```python
from build123d import *

# Parameters (mm, degrees)
SKETCH_1_W          = 9
SKETCH_1_H          = 9
EXTRUDE_1_DEPTH     = 3
SKETCH_2_W          = 14
SKETCH_2_H          = 14
EXTRUDE_2_DEPTH     = 2.5
CHAMFER_1_SIZE      = 1.5
SKETCH_3_W          = 12
SKETCH_3_H          = 10.4
EXTRUDE_3_DEPTH     = 12
EXTRUDE_4_DEPTH     = 2.3
SKETCH_5_W          = 0.5
SKETCH_5_H          = 3
EXTRUDE_5_DEPTH     = 4
SKETCH_6_W          = 1.2
SKETCH_6_H          = 2
CUT_EXTRUDE_1_DEPTH = 4


with BuildPart() as part:
    # Эскиз1 → Бобышка-Вытянуть1 (new body)
    with BuildSketch(Plane(origin=(0, 0, 0), x_dir=(1, 0, 0), z_dir=(0, 1, 0))):
        Rectangle(SKETCH_1_W, SKETCH_1_H)
    extrude(amount=EXTRUDE_1_DEPTH)

    # Эскиз2 → Бобышка-Вытянуть2 (add)
    with BuildSketch(Plane.XZ):
        Rectangle(SKETCH_2_W, SKETCH_2_H)
    extrude(amount=EXTRUDE_2_DEPTH)

    # Фаска1
    chamfer_1_edges = [part.edges().sort_by_distance(p)[0] for p in [
        (7, 0, 0),
        (0, 0, 7),
        (-7, 0, 0),
        (0, 0, -7),
    ]]
    chamfer(chamfer_1_edges, length=CHAMFER_1_SIZE)

    # Эскиз3 → Бобышка-Вытянуть3 (add)
    with BuildSketch(Plane.XZ.offset(2.5)):
        Rectangle(SKETCH_3_W, SKETCH_3_H)
    extrude(amount=EXTRUDE_3_DEPTH)

    # Эскиз4 → Бобышка-Вытянуть4 (add)
    with BuildSketch(Plane.XZ.offset(14.5)):
        Polygon((4.188675038, -1.5), (4.188675038, 1.5), (3.342315947, 2.5), (2.960661433, 2.176983233), (3.688675038, 1.316812163), (3.688675038, -1.316812163), (2.960661433, -2.176983233), (3.342315947, -2.5), align=None)
    extrude_4 = extrude(amount=EXTRUDE_4_DEPTH)

    # Эскиз5 → Бобышка-Вытянуть5 (add)
    with BuildSketch(Plane.XZ.offset(16.8)):
        with Locations((3.938675038, 0)):
            Rectangle(SKETCH_5_W, SKETCH_5_H)
    extrude_5 = extrude(amount=EXTRUDE_5_DEPTH)

    # Эскиз6 → Вырез-Вытянуть1 (cut)
    with BuildSketch(Plane.ZY.offset(-3.688675038)):
        with Locations((0, -18.8)):
            Rectangle(SKETCH_6_W, SKETCH_6_H)
    cut_extrude_1 = extrude(amount=-CUT_EXTRUDE_1_DEPTH, mode=Mode.SUBTRACT)

    # Зеркальное отражение1: Бобышка-Вытянуть4, Бобышка-Вытянуть5, Вырез-Вытянуть1 across plane
    add(extrude_4.mirror(Plane(origin=(0, 0, 0), x_dir=(0, 0, 1), z_dir=(1, 0, 0))))
    add(extrude_5.mirror(Plane(origin=(0, 0, 0), x_dir=(0, 0, 1), z_dir=(1, 0, 0))))
    add(cut_extrude_1.mirror(Plane(origin=(0, 0, 0), x_dir=(0, 0, 1), z_dir=(1, 0, 0))), mode=Mode.SUBTRACT)


solid = part.part
```
Can you work these out from the model? Positions are in its coordinate system, mm. A direction names the side the tool comes from. Round coordinates to 2 decimals unless told otherwise and drop trailing zeros. Order: outer loops, then holes, each group sorted by start corner. A loop starts at its lowest first (then second) coordinate and runs counter-clockwise, first axis right, second up. Notation, with made-up numbers: (60, 36.5) -> (100, 36.5) arc R34 ccw to (100, 68.5) -> close; hole circle Ø1 at (-17, 13). An arc over 180 degrees is marked (long way). Return JSON: item names as keys, results as strings. Group by question number.
1. If we section it at A-A, the plane z = 0: Count the separate pieces of the cut face and the enclosed holes in it, then the cut area to 3 significant figures.
2. If we section it at B-B, the plane y = -17.25: Write out the boundary of the cut face in (x, z), then the cut area to 3 significant figures.
3. We'd pull the mould along Z, two halves only. Please class faces 4 (the face through (-3.771, -15.634, 1.993)), 5 (the face through (3.32, -15.63, 1.75)), 6 (the face through (6.3, -0.8, -0.1)): released by +Z, released by -Z, zero draft, split by the parting line, or undercut.
4. Will these pins go through, and if not, where does the flat tip stop? pin 1 (0.9 mm diameter, centred on x = -3.5, z = -2, fed in from -Y); pin 2 (0.9 mm diameter, centred on y = 1, z = -0.5, fed in from +X); pin 3 (8 mm diameter, centred on y = -7.5, z = -2.5, fed in from +X); pin 4 (5 mm diameter, centred on x = 1.5, y = -3, fed in from -Z).
5. If we section it at D-D, the plane z = 4: Write out the boundary of the cut face in (x, y), then the cut area to 3 significant figures.
6. Which directions (+Z, -Z, +X, -X, +Y, -Y) give clear straight access to the entire face, cutting with the end or side of a thin tool? Please do faces 1 (the face through (4.5, 1, 0)), 2 (the face through (-3.33, -15.63, -1.74)), 3 (the face through (-3.76, -15.634, -2.007)).
7. I need wall thicknesses on line 1 (Z direction, x = -4.25, y = -8.75); line 2 (Y direction, x = -1.75, z = 3); line 3 (X direction, y = -7.5, z = -1). Which ranges of each line are inside material? Lowest first, please. Write a range as [from, to].
8. If we section it at C-C, the plane x = 5.75: Write out the boundary of the cut face in (y, z).
Output values:
{
 "1": {"separate pieces": "3", "enclosed holes": "0", "area": "208 mm²"},
 "2": {"outline": "(-4.19, -1.5) -> (-3.69, -1.5) -> (-3.69, 1.5) -> (-4.19, 1.5) -> close; (3.69, -1.5) -> (4.19, -1.5) -> (4.19, 1.5) -> (3.69, 1.5) -> close", "area": "3.00 mm²"},
 "3": {"face 4": "released by +Z", "face 5": "undercut", "face 6": "zero draft"},
 "4": {"pin 1": "y = -16.8", "pin 2": "x = 4.5", "pin 3": "x = 6", "pin 4": "z = -7"},
 "5": {"outline": "(-7, -2.5) -> (-6, -2.5) -> (-6, -14.5) -> (6, -14.5) -> (6, -2.5) -> (7, -2.5) -> (7, -1.5) -> (5.5, 0) -> (4.5, 0) -> (4.5, 3) -> (-4.5, 3) -> (-4.5, 0) -> (-5.5, 0) -> (-7, -1.5) -> close", "area": "204 mm²"},
 "6": {"face 1": "+Z, -Z, +X, +Y", "face 2": "-Y", "face 3": "-Z, -X, -Y"},
 "7": {"line 1": "[-5.2, 5.2]", "line 2": "[-14.5, 3]", "line 3": "[-6, 6]"},
 "8": {"outline": "(-14.5, -5.2) -> (-2.5, -5.2) -> (-2.5, -7) -> (-1.5, -7) -> (-0.25, -5.75) -> (-0.25, 5.75) -> (-1.5, 7) -> (-2.5, 7) -> (-2.5, 5.2) -> (-14.5, 5.2) -> close"}
}
